Work out the finished part from the listing and answer in its coordinate system (mm). A direction names the side the tool comes from. Round coordinates to 2 decimals unless told otherwise and drop trailing zeros. Loops run counter-clockwise (first coordinate to the right, second up) from the corner with the lowest first, then second, coordinate; pieces in that order, holes last. Notation, with made-up numbers: M 27.25,59 L 85.25,59 A20 ccw 85.25,85 Z; hole C -34.75,40.25 d6. An arc over 180 degrees is marked long. One line per item, written item: value.
```python
from build123d import *

# Parameters (mm, degrees)
MODEL_R         = 2.5999948
MODEL_R_2       = 2.0999958
EXTRUDE_1_DEPTH = 4


with BuildPart() as part:
    # Model → Бобышка-Вытянуть1 (new body)
    with BuildSketch(Plane.XY):
        with BuildLine():
            Line((308.392658055, 233.393719024), (308.392658055, 210.464832693))
            ThreePointArc((308.392658055, 210.464832693), (306.92819489, 206.929305859), (303.392668055, 205.464842693))
            Line((303.392668055, 205.464842693), (263.392748055, 205.464842693))
            ThreePointArc((263.392748055, 205.464842693), (259.85722122, 206.929305859), (258.392758055, 210.464832693))
            Line((258.392758055, 210.464832693), (258.392758055, 280.464692693))
            ThreePointArc((258.392758055, 280.464692693), (259.85722122, 284.000219528), (263.392748055, 285.464682693))
            Line((263.392748055, 285.464682693), (273.392728055, 285.464682693))
            ThreePointArc((273.392728055, 285.464682693), (276.92825489, 284.000219528), (278.392718055, 280.464692693))
            Line((278.392718055, 280.464692693), (278.392718055, 270.464712693))
            ThreePointArc((278.392718055, 270.464712693), (279.85718122, 266.929185859), (283.392708055, 265.464722693))
            Line((283.392708055, 265.464722693), (293.392688055, 265.464722693))
            ThreePointArc((293.392688055, 265.464722693), (296.92821489, 264.000259528), (298.392678055, 260.464732693))
            Line((298.392678055, 260.464732693), (298.392678055, 247.535826363))
            ThreePointArc((298.392678055, 247.535826363), (298.773279631, 245.622413028), (299.85714122, 244.000299528))
            Line((299.85714122, 244.000299528), (306.92819489, 236.929245859))
            ThreePointArc((306.92819489, 236.929245859), (308.012056479, 235.307132359), (308.392658055, 233.393719024))
        make_face()
        with Locations((286.392702055, 230.464792693)):
            Circle(MODEL_R, mode=Mode.SUBTRACT)
        with Locations((301.392672055, 215.464822693)):
            Circle(MODEL_R, mode=Mode.SUBTRACT)
        with Locations((268.392738055, 275.464702693)):
            Circle(MODEL_R_2, mode=Mode.SUBTRACT)
        with Locations((268.392738055, 247.464758693)):
            Circle(MODEL_R_2, mode=Mode.SUBTRACT)
        with Locations((288.392698055, 247.464758693)):
            Circle(MODEL_R_2, mode=Mode.SUBTRACT)
    extrude(amount=EXTRUDE_1_DEPTH)


solid = part.part
```
1) Find section A-A (x = 269.5). Give the vertices of the cut face in (y, z).
Check values:
outline: M 205.46,0 L 245.68,0 L 245.68,4 L 205.46,4 Z; M 249.25,0 L 273.68,0 L 273.68,4 L 249.25,4 Z; M 277.25,0 L 285.46,0 L 285.46,4 L 277.25,4 Z
2) Find the intervals of material crossed by probe 1 along Y at (x, z) = (270, 0.45); probe 2 along Y at (x, z) = (263, 2.85); probe 3 along Y at (x, z) = (303.5, 0.55), in increasing order. Write a range as from..to.
Check values:
probe 1: 205.46..246.11, 248.82..274.11, 276.82..285.46
probe 2: 205.48..285.45
probe 3: 205.47..213.94, 216.99..240.36
3) For faces 4 (the face through (278.393, 276, 2)), 5 (the face through (284, 205.465, 2)), determine the directions among +Z, -Z, +X, -X, +Y, -Y from which every point of the face is accessible in a straight line to the end or side of a thin tool.
Check values:
face 4: +Z, -Z, +X, +Y
face 5: +Z, -Z, +X, -X, -Y
4) Find section B-B (z = 1.4). Give the vertices of the cut face in (x, y).
Check values:
outline: M 258.39,210.46 A5 ccw 263.39,205.46 L 303.39,205.46 A5 ccw 308.39,210.46 L 308.39,233.39 A5 ccw 306.93,236.93 L 299.86,244 A5 cw 298.39,247.54 L 298.39,260.46 A5 ccw 293.39,265.46 L 283.39,265.46 A5 cw 278.39,270.46 L 278.39,280.46 A5 ccw 273.39,285.46 L 263.39,285.46 A5 ccw 258.39,280.46 Z; hole C 268.39,247.46 d4.2; hole C 268.39,275.46 d4.2; hole C 286.39,230.46 d5.2; hole C 288.39,247.46 d4.2; hole C 301.39,215.46 d5.2
5) The mould has two halves that part along Y. Classify faces 1 (the face through (298.393, 254, 2)), 2 (the face through (286.054, 233.043, 1.972)), 3 (the face through (259.82, 283.96, 1.97)): +Y half, -Y half, draft (parallel to the pull), parting line (faces both ways), or undercut.
Check values:
face 1: draft
face 2: undercut
face 3: +Y half
6) Find section C-C (y = 229). Give the vertices of the cut face in (x, z).
Check values:
outline: M 258.39,0 L 284.24,0 L 284.24,4 L 258.39,4 Z; M 288.54,0 L 308.39,0 L 308.39,4 L 288.54,4 Z
7) Find section D-D (y = 251.5). Give the vertices of the cut face in (x, z), then the cut area to 3 significant figures.
Check values:
outline: M 258.39,0 L 298.39,0 L 298.39,4 L 258.39,4 Z
area: 160 mm2
8) Each of these flat-tipped pins is pushed along its axis until it touches: pin 1 (4.5 mm diameter, centred on x = 286.39, y = 230.46, fed in from +Z); pin 2 (2 mm diameter, centred on x = 289.5, z = 2.5, fed in from +Y); pin 3 (2 mm diameter, centred on y = 245, z = 2.5, fed in from +X). Where does it stop, or does it pass through?
Check values:
pin 1: through
pin 2: y = 265.46
pin 3: x = 299.86
